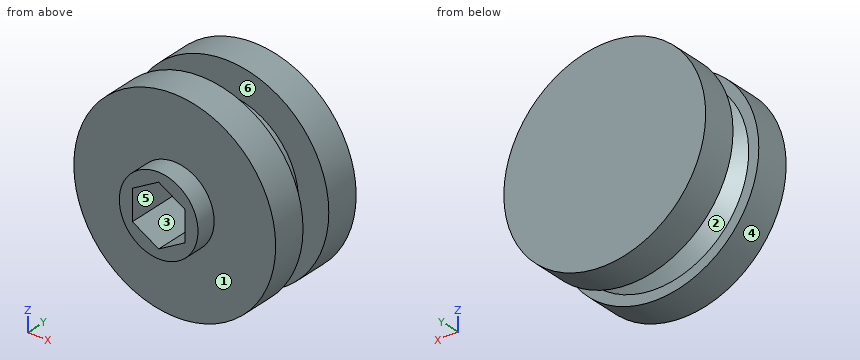
```python
from build123d import *

# Parameters (mm, degrees)
F3_DEPTH = 6
F4_SIZE2 = 1
F4_SIZE  = 2
F2_R     = 3.9
F5_DEPTH = 2


with BuildPart() as f1:
    # F0 (on Right) → F1 (revolve)
    with BuildSketch(Plane.YZ):
        Polygon((1.6, 6.9834658491), (0, 6.9834658491), (-1.6, 6.9834658491), (-1.6, 9.9834658491), (-5, 9.9834658491), (-5, -0.0165341509), (5, -0.0165341509), (5, 9.9834658491), (1.6, 9.9834658491), align=None)
    revolve(axis=Axis((0, 0, -0.0165341509), (0, 1, 0)))

    # F2 (on face) → F3 (cut)
    with BuildSketch(Plane.XZ.offset(5)):
        Polygon((2.6, -1.5011106999), (2.6, 1.5011106999), (0, 3.0022213998), (-2.6, 1.5011106999), (-2.6, -1.5011106999), (0, -3.0022213998), align=None)
    extrude(amount=-F3_DEPTH, mode=Mode.SUBTRACT)

    # F4
    f4_edges = [f1.edges().sort_by_distance(p)[0] for p in [
        (0, -1.6, -7.016534),
    ]]
    f4_side = f1.faces().sort_by_distance((0, -1.6, -7.299377))[0]
    chamfer(f4_edges, length=F4_SIZE, length2=F4_SIZE2, reference=f4_side)

    # F2 (on face) → F5 (join)
    with BuildSketch(Plane.XZ.offset(5)):
        Circle(F2_R)
        Polygon((0, 3.0022213998), (2.6, 1.5011106999), (2.6, -1.5011106999), (0, -3.0022213998), (-2.6, -1.5011106999), (-2.6, 1.5011106999), align=None, mode=Mode.SUBTRACT)
    extrude(amount=F5_DEPTH)


solid = f1.part
```
Source: CAD feature listing. Evaluate the final solid. Frame: model axes, mm. Face numbers are marked on the shaded views. A direction names the side the tool comes from. Round coordinates to 2 decimals unless told otherwise and drop trailing zeros. Write each loop counter-clockwise with the first axis right and the second up, starting at its lowest first coordinate (ties: lowest second). Pieces come first, ordered by that corner, then holes. Notation, with made-up numbers: M 26.5,47 L 84.5,47 A33 ccw 84.5,86 Z; hole C 15,50 d2. An arc over 180 degrees is marked long. Answer as a JSON object with one key per item and string values. Group by question number.
(1) Mould query, pull axis X, two halves, no side actions, for the marked faces 1, 2 and 3. Classes: +X half, -X half, draft (parallel to the pull), parting line (faces both ways), or undercut.
(2) First-contact query: pin 1 (3 mm diameter, centred on x = -3, y = 3.5, fed in from +Z); pin 2 (1 mm diameter, centred on y = -2.5, z = 1, fed in from +X); pin 3 (2 mm diameter, centred on y = -2.5, z = 6, fed in from -X). Flat tips, straight axial feed; report the tip coordinate or a pass-through.
(3) Ray query, line 1 (Y direction, x = 6.5, z = 6.25); line 2 (X direction, y = -0.5, z = 2.75); line 3 (Z direction, x = -1, y = -6.25). Return the intervals inside material, ascending. Write a range as [from, to].
(4) Reachability of the marked faces 4, 5 and 6 from +Z, -Z, +X, -X, +Y, -Y: full face, straight path, thin tool, end or side. Return the list, or none.
(5) Section query B-B on y = 3.5. Output: boundary loops of the cut face in (x, z).
(6) Section query A-A on y = -2.25. Output: boundary loops of the cut face in (x, z), then the cut area to 3 significant figures.
Computed values:
{
 "1": {"face 1": "draft", "face 2": "parting line", "face 3": "undercut"},
 "2": {"pin 1": "z = 9.87", "pin 2": "x = 9.99", "pin 3": "x = -8.65"},
 "3": {"line 1": "[-5, -1.6], [1.6, 5]", "line 2": "[-6.43, -0.44], [0.44, 6.43]", "line 3": "[-3.77, -2.42], [2.42, 3.77]"},
 "4": {"face 4": "+Y, -Y", "face 5": "-Y", "face 6": "none"},
 "5": {"outline": "C 0,-0.02 d20"},
 "6": {"outline": "C 0,-0.02 d20; hole M -2.6,-1.5 L 0,-3 L 2.6,-1.5 L 2.6,1.5 L 0,3 L -2.6,1.5 Z", "area": "291 mm^2"}
}
